For this review, take the finished solid that the model builds, in its own axes (mm). Face numbers are marked on the shaded views. A direction names the side the tool comes from. Round coordinates to 2 decimals unless told otherwise and drop trailing zeros. Loops run counter-clockwise (first coordinate to the right, second up) from the corner with the lowest first, then second, coordinate; pieces in that order, holes last. Notation, with made-up numbers: (28.5, 18.25) -> (56.5, 18.25) arc R16 cw to (56.5, 38.25) -> close; hole circle Ø4 at (84, 68.5). An arc over 180 degrees is marked (long way). One line per question, with ' | ' between items. Start each with the question number.
1. For pin 1 Ø6 at (x, y) = (8.5, -28.5) entering from -Z; pin 2 Ø8 at (x, z) = (0, -48.5) entering from +Y; pin 3 Ø7.5 at (x, z) = (-1, -23) entering from -Y, all flat-tipped, find the tip position at first contact; note any pin that passes through.
2. For the marked faces 4 and 5, list the 3-axis set-ups (+Z, -Z, +X, -X, +Y, -Y) from which the entire face can be reached by the end or side of a thin tool; tool diameter is ignored.
3. Wall thickness on line 1 along Y through (x, z) = (0, 3.25) (3 decimals); line 2 along X through (y, z) = (2.5, -12.7) (3 decimals); line 3 along Z through (x, y) = (-6, -35): over which ranges is each line inside the solid? List them lowest first.
4. Draft analysis for pull direction X (two halves, no side actions). For the marked faces 1, 2 and 3, state which applies: pulls with the +X half, pulls with the -X half, needs draft (parallel to the pull), parting line crosses it, or undercut.
5. Consider section D-D (x = -10). Write out the cut boundary in (y, z), and give its area (3 significant figures).
6. Consider section B-B (x = 0). Write out the cut boundary in (y, z) (3 decimals), and give its area (3 significant figures).
7. Consider section A-A (y = -19.05). Write out the cut boundary in (x, z) (3 decimals), and give its area (3 significant figures).
```python
from build123d import *

# Parameters (mm, degrees)
BOSS_EXTRUDE1_DEPTH = 12.7
SKETCH2_R           = 3.175
CUT_EXTRUDE1_DEPTH  = 100.595858348
SKETCH3_R           = 3.175
CUT_EXTRUDE2_DEPTH  = 100.595858348


with BuildPart() as part:
    # Sketch1 → Boss-Extrude1 (new, symmetric)
    with BuildSketch(Plane(origin=(0, 0, 0), x_dir=(0, 0, -1), z_dir=(1, 0, 0))):
        Polygon((0, 0), (0, -69.85), (-6.35, -69.85), (-6.35, 6.35), (69.85, 6.35), (69.85, 0), align=None)
    extrude(amount=BOSS_EXTRUDE1_DEPTH, both=True)

    # Sketch2 → Cut-Extrude1 (cut, through all)
    with BuildSketch(Plane(origin=(0, 0, 0), x_dir=(1, 0, 0), z_dir=(0, 1, 0))):
        with Locations(Location((0, 50.8, 0), (0, 0, 90))):
            Circle(SKETCH2_R)
        with Locations(Location((0, 12.7, 0), (0, 0, 90))):
            Circle(SKETCH2_R)
    extrude(amount=CUT_EXTRUDE1_DEPTH, mode=Mode.SUBTRACT)

    # Sketch3 → Cut-Extrude2 (cut, through all)
    with BuildSketch(Plane.XY):
        with Locations((0, -57.15)):
            Circle(SKETCH3_R)
        with Locations((0, -19.05)):
            Circle(SKETCH3_R)
    extrude(amount=CUT_EXTRUDE2_DEPTH, mode=Mode.SUBTRACT)


solid = part.part
```
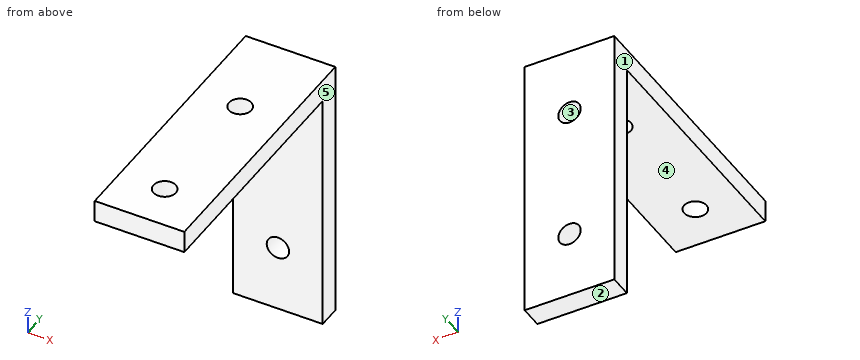
Answer block:
1) pin 1: stops at z = 0 | pin 2: stops at y = 6.35 | pin 3: stops at y = 0
2) face 4: -Z, +X, -X, -Y | face 5: +Z, -Z, +X, +Y, -Y
3) line 1: y = -69.85 to -60.325, -53.975 to -22.225, -15.875 to 6.35 | line 2: x = -12.7 to -3.175, 3.175 to 12.7 | line 3: z = 0 to 6.35
4) face 1: pulls with the -X half | face 2: needs draft | face 3: undercut
5) outline: (-69.85, 0) -> (0, 0) -> (0, -69.85) -> (6.35, -69.85) -> (6.35, 6.35) -> (-69.85, 6.35) -> close | area: 927 mm2
6) outline: (-69.85, 0) -> (-60.325, 0) -> (-60.325, 6.35) -> (-69.85, 6.35) -> close; (-53.975, 0) -> (-22.225, 0) -> (-22.225, 6.35) -> (-53.975, 6.35) -> close; (-15.875, 0) -> (0, 0) -> (0, -9.525) -> (6.35, -9.525) -> (6.35, 6.35) -> (-15.875, 6.35) -> close; (0, -69.85) -> (6.35, -69.85) -> (6.35, -53.975) -> (0, -53.975) -> close; (0, -47.625) -> (6.35, -47.625) -> (6.35, -15.875) -> (0, -15.875) -> close | area: 766 mm2
7) outline: (-12.7, 0) -> (-3.175, 0) -> (-3.175, 6.35) -> (-12.7, 6.35) -> close; (3.175, 0) -> (12.7, 0) -> (12.7, 6.35) -> (3.175, 6.35) -> close | area: 121 mm2
